Design review of the part built by this model. Coordinates are the model's own, in mm. A direction names the side the tool comes from. Coordinates: 2 decimals unless noted, no trailing zeros. Loops run counter-clockwise (first coordinate to the right, second up) from the corner with the lowest first, then second, coordinate; pieces in that order, holes last. Notation, with made-up numbers: (-16.5, -6.5) - (0.5, -6.5) arc R32 ccw to (0.5, 26.5) - close; hole circle Ø10 at (0, 45.25). An arc over 180 degrees is marked (long way). One line per question, with ' | ' between items.
Autodesk Inventor part; units mm, degrees
ref_plane "YZ Plane" through (0, 0, 0) normal (1, 0, 0) x (0, 1, 0)
ref_plane "XZ Plane" through (0, 0, 0) normal (0, 1, 0) x (-1, 0, 0)
ref_plane "XY Plane" through (0, 0, 0) normal (0, 0, 1) x (1, 0, 0)
sketch "Sketch2" plane through (0, 0, 0) normal (0, 0, 1) x (1, 0, 0)
  line L0 (0, 0) -> (200, 0) construction
  line L1 (200, 0) -> (200, 180) construction
  line L2 (200, 180) -> (0, 180) construction
  line L3 (0, 180) -> (0, 0) construction
  line L4 (0, 0) -> (75, 0) construction
  line L5 (75, 0) -> (125, 0)
  line L6 (125, 0) -> (200, 0) construction
  line L7 (0, 180) -> (0, 165)
  line L8 (200, 180) -> (200, 165)
  line L9 (200, 165) -> (125, 0)
  line L10 (75, 0) -> (0, 165)
  line L11 (0, 180) -> (8, 180)
  line L12 (200, 180) -> (192, 180)
  line L13 (119.8487, 8) -> (80.1513, 8)
  line L14 (8, 166.7329) -> (39.8628, 96.6347)
  line L15 (192, 166.7329) -> (160.1372, 96.6347)
  line L16 (160.1372, 96.6347) -> (39.8628, 96.6347)
  line L17 (8, 166.7329) -> (8, 180)
  line L18 (192, 166.7329) -> (192, 180)
  line L19 (42.1356, 91.6347) -> (80.1513, 8)
  line L20 (157.8644, 91.6347) -> (119.8487, 8)
  line L21 (42.1356, 91.6347) -> (157.8644, 91.6347)
  dimension "d0" = 200
  dimension "d1" = 180
  dimension "d2" = 75
  dimension "d3" = 50
  dimension "d4" = 15
  dimension "d5" = 15
  dimension "d6" = 8
  dimension "d7" = 8
  dimension "d10" = 77
  dimension "d11" = 8
  dimension "d12" = 8
  dimension "d14" = 8
  dimension "d15" = 5
extrude "Extrusion1" add sketch "Sketch2" along normal blind 20
fillet "Fillet1" radius 3 16 edges at (8, 180, 10) (0, 180, 10) (8, 166.7329, 10) (0, 165, 10) (200, 180, 10) (192, 180, 10) (200, 165, 10) (192, 166.7329, 10) (39.8628, 96.6347, 10) (42.1356, 91.6347, 10) (160.1372, 96.6347, 10) (157.8644, 91.6347, 10) (80.1513, 8, 10) (119.8487, 8, 10) (125, 0, 10) (75, 0, 10)
sketch "Sketch5" plane through (46.7946, 91.6347, 20) normal (0, -1, 0) x (1, 0, 0)
  line L0 (106.4109, -20) -> (0, -20)
  line L1 (0, -20) -> (0, 0)
  point P0 (-46.7946, -20)
  point P1 (40.2055, -10)
  point P2 (41.2055, -10)
  point P3 (59.2055, -10)
  point P4 (66.2055, -10)
  dimension "d39" = 1
  dimension "d40" = 18
  dimension "d41" = 7
  dimension "d42" = 10
  dimension "d43" = 40.2055
hole "Hole1" at (87.0001, 91.6347, 10) at (88.0001, 91.6347, 10) at (106.0001, 91.6347, 10) at (113.0001, 91.6347, 10) direction (0, -1, 0) diameter 3.5 end through all
sketch "Sketch6" plane through (76.9317, 0, 0) normal (0, -1, 0) x (1, 0, 0)
  arc A0 (10.5683, 11.6771) -> (10.5683, 8.3229) centre (10.0683, 10) ccw
  line L0 (10.0683, 11.75) -> (11.0683, 11.75)
  line L1 (10.0683, 8.25) -> (11.0683, 8.25)
  arc A1 (10.5683, 8.3229) -> (10.5683, 11.6771) centre (11.0683, 10) ccw
  point P0 (-76.9317, 0)
extrude "Extrusion2" cut sketch "Sketch6" against normal blind 8 contours A0 L0 A1 | A0 A1 L1
properties part number "PatasColaTrasera"
Q1. Tool access review of faces 1 (the flat face through (176.55, 132.74, 9.86)), 2 (the flat face through (0, 171, 10)), 3 (the flat face through (99, 91.635, 10)): name each direction out of +Z, -Z, +X, -X, +Y, -Y from which nothing blocks a thin tool from reaching the whole face with its end or side.
Returned:
face 1: +Z, -Z, +Y | face 2: +Z, -Z, -X, +Y, -Y | face 3: +Z, -Z
Q2. Take a section at C-C (x = 144.5). Give the boundary of the cut face in (y, z).
Returned:
outline: (42.9, 0) - (62.23, 0) - (62.23, 20) - (42.9, 20) - close; (91.63, 0) - (96.63, 0) - (96.63, 20) - (91.63, 20) - close
Q3. To check wall thickness, follow line 1 along Y through (x, z) = (112.5, 1.75); line 2 along X through (y, z) = (2.5, 10); line 3 along X through (y, z) = (5.25, 10). State the ranges of each line that lie inside material, in increasing order.
Returned:
line 1: y = 0 to 8, 91.63 to 96.63 | line 2: x = 73.86 to 85.25, 89.75 to 104.25, 107.75 to 111.25, 114.75 to 126.14 | line 3: x = 72.61 to 85.25, 89.75 to 104.25, 107.75 to 111.25, 114.75 to 127.39
Q4. Take a section at D-D (x = 185.5). Give the boundary of the cut face in (y, z), plus the area to 3 significant figures.
Returned:
outline: (133.1, 0) - (152.43, 0) - (152.43, 20) - (133.1, 20) - close | area: 387 mm²
Q5. For pin 1 (12 mm diameter, centred on y = 71.5, z = 2, fed in from +X); pin 2 (1 mm diameter, centred on y = 48, z = 12.5, fed in from -X); pin 3 (1.5 mm diameter, centred on x = 42.5, z = 14, fed in from -Y), all flat-tipped, find the tip position at first contact; note any pin that passes through.
Returned:
pin 1: stops at x = 160.23 | pin 2: stops at x = 52.95 | pin 3: stops at y = 69.85
Q6. Draft analysis for pull direction X (two halves, no side actions). For faces 4 (the flat face through (144, 57, 0)), 5 (the flat face through (8, 172, 10)), 6 (the flat face through (200, 171, 10)), state which applies: +X half, -X half, draft (parallel to the pull), parting line (faces both ways), or undercut.
Returned:
face 4: draft | face 5: undercut | face 6: +X half
Q7. Take a section at B-B (y = 80). Give the boundary of the cut face in (x, z).
Returned:
outline: (38.64, 0) - (47.42, 0) - (47.42, 20) - (38.64, 20) - close; (152.58, 0) - (161.36, 0) - (161.36, 20) - (152.58, 20) - close
